Source: CAD feature listing. Evaluate the final solid. Frame: model axes, mm. Give positions to 0.01 mm unless a question says otherwise; leave off trailing zeros. Order: outer loops, then holes, each group sorted by start corner. A loop starts at its lowest first (then second) coordinate and runs counter-clockwise, first axis right, second up. Notation, with made-up numbers: (-15, -34) -> (3, -34) arc R11 ccw to (3, -26) -> close; hole circle Ø1 at (65.25, 88). An arc over 180 degrees is marked (long way). Answer in a Markdown table with one row per item.
```python
from build123d import *

# Parameters (mm, degrees)
SKETCH_1_R        = 1.3
EXTRUDE_127_DEPTH = 1.2


with BuildPart() as part:
    # 草图1 → 柔性桨叶包络_展开总径127 (new body)
    with BuildSketch(Plane.XY):
        Polygon((-3, -3), (3, -4), (12, -7), (30, -9), (44, -5), (55.5, -1), (54, 3), (36, 4), (18, 3), (4, 3), (-3, 3), align=None)
        Circle(SKETCH_1_R, mode=Mode.SUBTRACT)
    extrude(amount=EXTRUDE_127_DEPTH)


solid = part.part
```
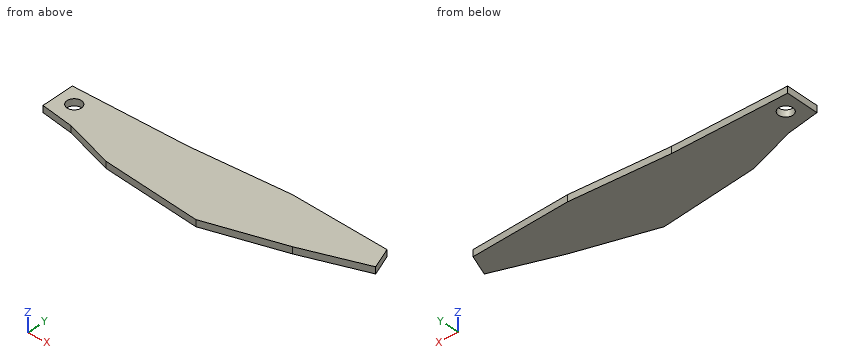
(1) Section query B-B (y = 0.75). Return the cut outline in (x, z), plus the area to 3 significant figures.
A:
| item | result |
|---|---|
| outline | (-3, 0) -> (-1.06, 0) -> (-1.06, 1.2) -> (-3, 1.2) -> close; (1.06, 0) -> (54.84, 0) -> (54.84, 1.2) -> (1.06, 1.2) -> close |
| area | 66.9 mm^2 |
(2) Section query A-A (x = 0). Return the cut outline in (y, z), plus the area to 3 significant figures.
A:
| item | result |
|---|---|
| outline | (-3.5, 0) -> (-1.3, 0) -> (-1.3, 1.2) -> (-3.5, 1.2) -> close; (1.3, 0) -> (3, 0) -> (3, 1.2) -> (1.3, 1.2) -> close |
| area | 4.68 mm^2 |
(3) Section query D-D (x = 45). Return the cut outline in (y, z), plus the area to 3 significant figures.
A:
| item | result |
|---|---|
| outline | (-4.65, 0) -> (3.5, 0) -> (3.5, 1.2) -> (-4.65, 1.2) -> close |
| area | 9.78 mm^2 |
(4) Section query C-C (z = 0.8). Return the cut outline in (x, y), plus the area to 3 significant figures.
A:
| item | result |
|---|---|
| outline | (-3, -3) -> (3, -4) -> (12, -7) -> (30, -9) -> (44, -5) -> (55.5, -1) -> (54, 3) -> (36, 4) -> (18, 3) -> (-3, 3) -> close; hole circle Ø2.6 at (0, 0) |
| area | 532 mm^2 |
(5) Ray query, probe 1 along Y at (x, z) = (0, 0.65); probe 2 along Y at (x, z) = (31, 0.7); probe 3 along Y at (x, z) = (36, 0.2). Return the intervals inside material, ascending.
A:
| item | result |
|---|---|
| probe 1 | y = -3.5 to -1.3, 1.3 to 3 |
| probe 2 | y = -8.71 to 3.72 |
| probe 3 | y = -7.29 to 4 |
